```python
from build123d import *

# Parameters (mm, degrees)
BOSS_EXTRUDE1_DEPTH = 48
SKETCH2_R           = 1.25
CUT_EXTRUDE1_DEPTH  = 66.639750601


with BuildPart() as part:
    # Sketch1 → Boss-Extrude1 (new body)
    with BuildSketch(Plane.XY):
        with BuildLine():
            Line((7.5, -21.990381057), (22.5, -21.990381057))
            ThreePointArc((22.5, -21.990381057), (27, -20.784609691), (30.294228634, -17.490381057))
            Line((30.294228634, -17.490381057), (37.794228634, -4.5))
            ThreePointArc((37.794228634, -4.5), (37.794228634, 4.5), (30, 9))
            Line((30, 9), (0, 9))
            ThreePointArc((0, 9), (-7.794228634, 4.5), (-7.794228634, -4.5))
            Line((-7.794228634, -4.5), (-0.294228634, -17.490381057))
            ThreePointArc((-0.294228634, -17.490381057), (3, -20.784609691), (7.5, -21.990381057))
        make_face()
        with BuildLine():
            ThreePointArc((3.75, -6.495190528), (3.75, -19.485571585), (15, -12.990381057))
            ThreePointArc((15, -12.990381057), (26.25, -19.485571585), (26.25, -6.495190528))
            ThreePointArc((26.25, -6.495190528), (36.495190528, 3.75), (22.5, 0))
            ThreePointArc((22.5, 0), (15, 7.5), (7.5, 0))
            ThreePointArc((7.5, 0), (-6.495190528, 3.75), (3.75, -6.495190528))
        make_face(mode=Mode.SUBTRACT)
    extrude(amount=BOSS_EXTRUDE1_DEPTH)

    # Sketch2 → Cut-Extrude1 (cut, through all)
    with BuildSketch(Plane(origin=(0, 0, 0), x_dir=(-1, 0, 0), z_dir=(0, 0, -1))):
        with Locations((1.576056233, -9.570190528)):
            Circle(SKETCH2_R)
        with Locations((-31.574981029, -9.570190528)):
            Circle(SKETCH2_R)
    extrude(amount=-CUT_EXTRUDE1_DEPTH, mode=Mode.SUBTRACT)


solid = part.part
```
The listing builds one solid part. Answer for the finished solid, in the listing's coordinates (mm). Round coordinates to 2 decimals unless told otherwise and drop trailing zeros. Loops run counter-clockwise (first coordinate to the right, second up) from the corner with the lowest first, then second, coordinate; pieces in that order, holes last. Notation, with made-up numbers: (-34.75, -37.75) - (2.25, -37.75) arc R22 ccw to (2.25, -2.75) - close; hole circle Ø1 at (-19, -0.75). An arc over 180 degrees is marked (long way). Use one line per item in the form item = value. Start each with the question number.
1. Given pin 1 Ø5 at (y, z) = (-10, 32.5) entering from +X; pin 2 Ø2 at (y, z) = (1.5, 32.5) entering from +X; pin 3 Ø8 at (y, z) = (-14.5, 24.5) entering from +X, each flat-ended and moving along its own axis, determine where each tip first touches the part or whether it passes through.
2. The part is cut by section A-A on x = 29. Determine the outline of the cut face in (y, z).
3. Consider line 1 (Y direction, x = 28, z = 41); line 2 (Y direction, x = 28.5, z = 39.5); line 3 (X direction, y = -17.5, z = 14.5). Determine where each line is inside the solid, lowest interval first. Write a range as [from, to].
4. The part is cut by section C-C on z = 13.5. Determine the outline of the cut face in (x, y), then the cut area to 3 significant figures.
5. For a pull along X with two mould halves and no side action, classify faces 1 (the face through (37.859, 4.385, 23.664)), 2 (the face through (2.94, -20.75, 23.66)), 3 (the face through (15, 9, 24)), 4 (the face through (15.16, 7.5, 23.66)) as pulls with the +X half, pulls with the -X half, needs draft (parallel to the pull), parting line crosses it, or undercut.
6. The part is cut by section B-B on y = -5.5. Determine the outline of the cut face in (x, z).
7. The part is cut by section D-D on y = 2. Determine the outline of the cut face in (x, z), then the cut area to 3 significant figures.
Geometry check:
q1.pin_1 = 36.06
q1.pin_2 = 38.99
q1.pin_3 = 34.33
q2.outline = (-19.22, 0) - (-16.73, 0) - (-16.73, 48) - (-19.22, 48) - close; (-9.25, 0) - (-7.43, 0) - (-7.43, 48) - (-9.25, 48) - close; (7.43, 0) - (9, 0) - (9, 48) - (7.43, 48) - close
q3.line_1 = [-20.11, -18.09], [-7.89, -7.23], [7.23, 9]
q3.line_2 = [-19.7, -17.49], [-8.49, -7.35], [7.35, 9]
q3.line_3 = [-0.29, 1.51], [13.49, 16.51], [28.49, 30.29]
q4.outline = (-7.79, -4.5) - (-0.29, -17.49) arc R9 ccw to (7.5, -21.99) - (22.5, -21.99) arc R9 ccw to (30.29, -17.49) - (37.79, -4.5) arc R9 ccw to (30, 9) - (0, 9) arc R9 ccw to start; hole circle Ø2.5 at (-1.58, -9.57); hole (3.75, -6.5) arc R7.5 ccw (long way) to (15, -12.99) arc R7.5 ccw (long way) to (26.25, -6.5) arc R7.5 ccw (long way) to (22.5, 0) arc R7.5 ccw to (7.5, 0) arc R7.5 ccw (long way) to start; hole circle Ø2.5 at (31.57, -9.57)
q4.area = 301 mm^2
q5.face_1 = pulls with the +X half
q5.face_2 = pulls with the -X half
q5.face_3 = needs draft
q5.face_4 = undercut
q6.outline = (-7.22, 0) - (-5.1, 0) - (-5.1, 48) - (-7.22, 48) - close; (35.1, 0) - (37.22, 0) - (37.22, 48) - (35.1, 48) - close
q7.outline = (-8.77, 0) - (-7.23, 0) - (-7.23, 48) - (-8.77, 48) - close; (7.23, 0) - (7.77, 0) - (7.77, 48) - (7.23, 48) - close; (22.23, 0) - (22.77, 0) - (22.77, 48) - (22.23, 48) - close; (37.23, 0) - (38.77, 0) - (38.77, 48) - (37.23, 48) - close
q7.area = 201 mm^2
